Read the model definition and answer for the solid it produces. Units are mm, in the model's axes. A direction names the side the tool comes from. Give positions to 0.01 mm unless a question says otherwise; leave off trailing zeros. Loops run counter-clockwise (first coordinate to the right, second up) from the corner with the lowest first, then second, coordinate; pieces in that order, holes last. Notation, with made-up numbers: (57.5, 56) -> (65.5, 56) arc R14 cw to (65.5, 62) -> close; hole circle Ø2 at (-26.5, -8.5). An arc over 180 degrees is marked (long way). Answer as CSV lines item,"result". Start each with the question number.
```python
from build123d import *

# Parameters (mm, degrees)
F0_R     = 25
F1_DEPTH = 50
F2_R     = 15
F3_DEPTH = 10
F4_W     = 80
F4_H     = 60
F5_DEPTH = 100


with BuildPart() as f1:
    # F0 (on Top) → F1 (new body, symmetric)
    with BuildSketch(Plane.XY):
        with BuildLine():
            Line((0, 50), (-50, 50))
            ThreePointArc((-50, 50), (-100, 0), (-50, -50))
            Line((-50, -50), (0, -50))
            Line((0, -50), (0, 50))
        make_face()
        with Locations((-50, 0)):
            Circle(F0_R, mode=Mode.SUBTRACT)
    extrude(amount=F1_DEPTH, both=True)

    # F2 (on Front) → F3 (join, symmetric)
    with BuildSketch(Plane.XZ):
        with BuildLine():
            Line((0, -50), (50, -50))
            ThreePointArc((50, -50), (100, 0), (50, 50))
            Line((50, 50), (0, 50))
            Line((0, 50), (0, -50))
        make_face()
        with Locations((50, 0)):
            Circle(F2_R, mode=Mode.SUBTRACT)
    extrude(amount=F3_DEPTH, both=True)

    # F4 (on Front) → F5 (cut, symmetric)
    with BuildSketch(Plane.XZ):
        with Locations((-60, 0)):
            Rectangle(F4_W, F4_H)
    extrude(amount=F5_DEPTH, both=True, mode=Mode.SUBTRACT)


solid = f1.part
```
(1) The mould has two halves that part along X. Classify faces 6 (the face through (-70, -15, -40)), 7 (the face through (-70, -15, 40)), 8 (the face through (0, -30, 1)), 9 (the face through (-19, 50, 1)): pulls with the +X half, pulls with the -X half, needs draft (parallel to the pull), parting line crosses it, or undercut.
(2) Find section C-C on z = -2. Write down the section's boundary in (x, y).
(3) Find section A-A on y = 0. Write down the section's boundary in (x, z), then the cut area to 3 significant figures.
(4) A tool of negligible diameter and unlimited length cuts with its end or side. For faces 1 (the face through (-78, -1, -30)), 2 (the face through (-19.8, -50, 0.7)), 3 (the face through (99.988, -0.14, -1.099)), 4 (the face through (38, -10, -10)), 5 (the face through (38, 10, -10)), from which of +Z, -Z, +X, -X, +Y, -Y can it reach the whole face along a straight path? Write none if from no direction.
(5) Each of these flat-tipped pins is pushed along its axis until it touches: P1, Ø5, axis at y = 32, z = -39, coming from the +X side; P2, Ø3, axis at x = -61, y = 21, coming from the +Z side; P3, Ø8, axis at y = -38.5, z = 37.5, coming from the -X side. Where does it stop, or does it pass through?
(6) Find section D-D on y = 40. Write down the section's boundary in (x, z).
(7) Find section B-B on x = 45.5. Write down the section's boundary in (y, z).
(8) Find the intervals of material crossed by line 1 along Y through (x, z) = (-50, -44.25); line 2 along Z through (x, y) = (50, 1); line 3 along Z through (x, y) = (-78, 3), in increasing order. Write a range as from..to.
Answer block:
1,face 6,"undercut"
1,face 7,"undercut"
1,face 8,"pulls with the +X half"
1,face 9,"needs draft"
2,outline,"(-20, -50) -> (0, -50) -> (0, -10) -> (35.13, -10) -> (35.13, 10) -> (0, 10) -> (0, 50) -> (-20, 50) -> close; (64.87, -10) -> (99.96, -10) -> (99.96, 10) -> (64.87, 10) -> close"
3,outline,"(-100, -50) -> (-75, -50) -> (-75, -30) -> (-100, -30) -> close; (-100, 30) -> (-75, 30) -> (-75, 50) -> (-100, 50) -> close; (-25, -50) -> (50, -50) arc R50 ccw to (50, 50) -> (-25, 50) -> (-25, 30) -> (-20, 30) -> (-20, -30) -> (-25, -30) -> close; hole circle Ø30 at (50, 0)"
3,area,"11,400 mm2"
4,face 1,"-X, +Y, -Y"
4,face 2,"+Z, -Z, +X, -X, -Y"
4,face 3,"+X, +Y, -Y"
4,face 4,"+Z, -Z, +X, -Y"
4,face 5,"+Z, -Z, +X, +Y"
5,P1,"stops at x = 0"
5,P2,"stops at z = 50"
5,P3,"stops at x = -86.19"
6,outline,"(-80, -50) -> (0, -50) -> (0, 50) -> (-80, 50) -> (-80, 30) -> (-20, 30) -> (-20, -30) -> (-80, -30) -> close"
7,outline,"(-10, -50) -> (10, -50) -> (10, -14.31) -> (-10, -14.31) -> close; (-10, 14.31) -> (10, 14.31) -> (10, 50) -> (-10, 50) -> close"
8,line 1,"y = -50..-25, 25..50"
8,line 2,"z = -50..-15, 15..50"
8,line 3,"z = -50..-30, 30..50"
